Source: CAD feature listing. Evaluate the final solid. Frame: model axes, mm. A direction names the side the tool comes from. Give positions to 0.01 mm unless a question says otherwise; leave off trailing zeros. Write each loop counter-clockwise with the first axis right and the second up, starting at its lowest first coordinate (ties: lowest second). Pieces come first, ordered by that corner, then holes. Notation, with made-up numbers: M 29.5,56.25 L 76.5,56.25 A17 cw 76.5,73.25 Z; hole C -29.75,64.5 d8. An arc over 180 degrees is marked long. Return JSON: item names as keys, results as strings.
```python
from build123d import *

# Parameters (mm, degrees)
SKETCH1_W                       = 19.05
SKETCH1_H                       = 101.6
BOSS_EXTRUDE1_DEPTH             = 9.525
SKETCH2_W                       = 6.35
SKETCH2_H                       = 9.525
CUT_EXTRUDE1_DEPTH              = 103.489078686
F_1_4_0_25_DIAMETER_HOLE1_D     = 6.35
F_1_4_0_25_DIAMETER_HOLE1_DEPTH = 25.4
F_1_4_0_25_DIAMETER_HOLE1_TIP   = 1.907732465


with BuildPart() as part:
    # Sketch1 → Boss-Extrude1 (new, symmetric)
    with BuildSketch(Plane(origin=(0, 0, 0), x_dir=(1, 0, 0), z_dir=(0, 1, 0))):
        Rectangle(SKETCH1_W, SKETCH1_H)
    extrude(amount=BOSS_EXTRUDE1_DEPTH, both=True)

    # Sketch2 → Cut-Extrude1 (cut, through all)
    with BuildSketch(Plane.XY.offset(50.8)):
        with Locations((6.35, -4.7625)):
            Rectangle(SKETCH2_W, SKETCH2_H)
    extrude(amount=-CUT_EXTRUDE1_DEPTH, mode=Mode.SUBTRACT)

    # 1/4 (0.25) Diameter Hole1
    with Locations(Plane(origin=(0, 9.525, 0), x_dir=(1, 0, 0), z_dir=(0, 1, 0))):
        with Locations((-3.175, 31.75), (-3.175, -31.75)):
            Hole(F_1_4_0_25_DIAMETER_HOLE1_D / 2, depth=F_1_4_0_25_DIAMETER_HOLE1_DEPTH)
            with Locations((0, 0, -(F_1_4_0_25_DIAMETER_HOLE1_DEPTH + F_1_4_0_25_DIAMETER_HOLE1_TIP / 2))):  # 118° drill point
                Cone(0, F_1_4_0_25_DIAMETER_HOLE1_D / 2, F_1_4_0_25_DIAMETER_HOLE1_TIP, mode=Mode.SUBTRACT)


solid = part.part
```
1) Cut plane B-B, the plane z = -31.75. Return the cut outline in (x, y) (3 decimals).
Numbers:
{"outline": "M -9.525,-9.525 L -6.35,-9.525 L -6.35,9.525 L -9.525,9.525 Z; M 0,-9.525 L 3.175,-9.525 L 3.175,0 L 9.525,0 L 9.525,9.525 L 0,9.525 Z"}
2) Contact query for flat-ended pins moving along their axis: pin 1 Ø5 at (y, z) = (-4.5, 15.5) entering from +X (3 decimals); pin 2 Ø5 at (x, z) = (5.5, -7.5) entering from -Y (3 decimals); pin 3 Ø1.5 at (x, z) = (6, 27) entering from -Y. Output: stop coordinate, or through.
Numbers:
{"pin 1": "stops at x = 3.175", "pin 2": "stops at y = -9.525", "pin 3": "stops at y = 0"}
3) Set-up query: faces 1 (the face through (3.175, -5, 1)), 2 (the face through (-2, 0, 50.8)). Return all of +Z, -Z, +X, -X, +Y, -Y with unobstructed straight access to the full face (end or side cutting, diameter ignored); none if empty.
Numbers:
{"face 1": "+Z, -Z, +X, -Y", "face 2": "+Z, +X, -X, +Y, -Y"}
4) Cut plane A-A, the plane y = -4.75. Return the cut outline in (x, z) (3 decimals), then the cut area to 3 significant figures.
Numbers:
{"outline": "M -9.525,-50.8 L 3.175,-50.8 L 3.175,50.8 L -9.525,50.8 Z; hole C -3.175,-31.75 d6.35; hole C -3.175,31.75 d6.35", "area": "1,230 mm²"}
5) Line query: line 1 (X direction, y = -4, z = -31.75) (3 decimals); line 2 (Z direction, x = -5.5, y = 7.5); line 3 (Z direction, x = -1.75, y = 4). Output: solid intervals per line, ascending. Write a range as [from, to].
Numbers:
{"line 1": "x = [-9.525, -6.35], [0, 3.175]", "line 2": "z = [-50.8, -33.91], [-29.59, 29.59], [33.91, 50.8]", "line 3": "z = [-50.8, -34.59], [-28.91, 28.91], [34.59, 50.8]"}
6) Draft query along Z for faces 3 (the face through (6, 0, 1)), 4 (the face through (-2.49, -0.13, 34.85)), 5 (the face through (-2, 0, -50.8)). Return one class per face: released by +Z, released by -Z, zero draft, split by the parting line, or undercut.
Numbers:
{"face 3": "zero draft", "face 4": "undercut", "face 5": "released by -Z"}
7) Cut plane D-D, the plane z = -17. Return the cut outline in (x, y) (3 decimals), then the cut area to 3 significant figures.
Numbers:
{"outline": "M -9.525,-9.525 L 3.175,-9.525 L 3.175,0 L 9.525,0 L 9.525,9.525 L -9.525,9.525 Z", "area": "302 mm²"}
8) Cut plane C-C, the plane x = -3.75. Return the cut outline in (y, z) (1 decimal), then the cut area to 3 significant figures.
Numbers:
{"outline": "M -9.5,-50.8 L 9.5,-50.8 L 9.5,-34.9 L -9.5,-34.9 Z; M -9.5,-28.6 L 9.5,-28.6 L 9.5,28.6 L -9.5,28.6 Z; M -9.5,34.9 L 9.5,34.9 L 9.5,50.8 L -9.5,50.8 Z", "area": "1,700 mm²"}
